For this review, take the finished solid that the model builds, in its own axes (mm). A direction names the side the tool comes from. Round coordinates to 2 decimals unless told otherwise and drop trailing zeros. Loops run counter-clockwise (first coordinate to the right, second up) from the corner with the lowest first, then second, coordinate; pieces in that order, holes last.
1) Take a section at D-D (y = 73.5). State the section outline as (x, z) points (3 decimals), then the cut area to 3 significant figures.
2) Take a section at A-A (y = 19). State the section outline as (x, z) points (3 decimals).
3) Take a section at B-B (x = -4). State the section outline as (y, z) points (3 decimals).
4) Mouldability with a two-part tool opening along Y and no side actions: class faces 4 (the flat face through (-31.75, -1, 283)), 5 (the flat face through (0.622, -246.174, -9.658)), 6 (the flat face through (1, 3, -9.525)), 7 (the flat face through (0.62, -240.94, -17.35)) as pulls with the +Y half, pulls with the -Y half, needs draft (parallel to the pull), parting line crosses it, or undercut.
5) Tool access review of faces 1 (the flat face through (0.622, 241.128, -17.574)), 2 (the flat face through (31.75, 1, 283)), 3 (the flat face through (0, 57.15, 275)): name each direction out of +Z, -Z, +X, -X, +Y, -Y from which nothing blocks a thin tool from reaching the whole face with its end or side.
6) Insertion check: pin 1 (10 mm diameter, centred on x = -3, z = 294, fed in from -Y); pin 2 (1.5 mm diameter, centred on y = 28, z = 144.5, fed in from -X); pin 3 (12 mm diameter, centred on x = -33, z = 262, fed in from +Y). Each pin has a flat end and moves straight along its axis. Give the tip position at first contact, or say it passes through.
7) Wall thickness on L1, parallel to Z at x = 18.5, y = -20 (3 decimals); L2, parallel to Z at x = -0.5, y = 86.5 (3 decimals); L3, parallel to X at y = 34, z = 45: over which ranges is each line inside the solid? List them lowest first.
8) Take a section at C-C (z = 388). State the section outline as (x, y) points.
```python
from build123d import *

# Parameters (mm, degrees)
F0_W      = 63.5
F0_H      = 114.3
F1_DEPTH  = 558.8
F2_SIZE   = 5.08
F4_DEPTH  = 25.4
F6_DEPTH  = 76.2
F8_DEPTH  = 12.7
F10_DEPTH = 12.7


with BuildPart() as f1:
    # F0 (on Top) → F1 (new body)
    with BuildSketch(Plane.XY):
        Rectangle(F0_W, F0_H)
    extrude(amount=F1_DEPTH)

    # F2
    f2_edges = [f1.edges().sort_by_distance(p)[0] for p in [
        (31.75, 57.15, 279.4),
        (-31.75, 57.15, 279.4),
        (-31.75, -57.15, 279.4),
        (31.75, -57.15, 279.4),
    ]]
    chamfer(f2_edges, length=F2_SIZE)

    # F3 (on face) → F4 (join)
    with BuildSketch(Plane(origin=(0, 0, 0), x_dir=(1, 0, 0), z_dir=(0, 0, -1))):
        Polygon((31.75, 52.07), (31.75, 254), (-31.75, 254), (-31.75, 52.07), (-26.67, 57.15), (26.67, 57.15), align=None)
        Polygon((31.75, -52.07), (31.75, 52.07), (26.67, 57.15), (-26.67, 57.15), (-31.75, 52.07), (-31.75, -52.07), (-26.67, -57.15), (26.67, -57.15), align=None)
        Polygon((31.75, -254), (31.75, -52.07), (26.67, -57.15), (-26.67, -57.15), (-31.75, -52.07), (-31.75, -254), align=None)
    extrude(amount=F4_DEPTH)

    # F5 (on face) → F6 (cut)
    with BuildSketch(Plane(origin=(-31.75, 0, 0), x_dir=(0, -1, 0), z_dir=(-1, 0, 0))):
        Polygon((238.125, 0), (254, -19.05), (254, 0), align=None)
        Polygon((-247.65, -25.4), (247.65, -25.4), (234.420833, -9.525), (-234.420833, -9.525), align=None)
        Polygon((-254, 0), (-254, -19.05), (-238.125, 0), align=None)
    extrude(amount=-F6_DEPTH, mode=Mode.SUBTRACT)

    # F7 (on face) → F8 (join)
    with BuildSketch(Plane.YZ.offset(31.75)):
        Polygon((238.125, 0), (52.07, 0), (-52.07, 0), (-238.125, 0), (-254, -19.05), (-254, -25.4), (-247.65, -25.4), (-234.420833, -9.525), (234.420833, -9.525), (247.65, -25.4), (254, -25.4), (254, -19.05), align=None)
    extrude(amount=F8_DEPTH)

    # F9 (on face) → F10 (join)
    with BuildSketch(Plane(origin=(-31.75, 0, 0), x_dir=(0, -1, 0), z_dir=(-1, 0, 0))):
        Polygon((238.125, 0), (52.07, 0), (-52.07, 0), (-238.125, 0), (-254, -19.05), (-254, -25.4), (-247.65, -25.4), (-234.420833, -9.525), (234.420833, -9.525), (247.65, -25.4), (254, -25.4), (254, -19.05), align=None)
    extrude(amount=F10_DEPTH)


solid = f1.part
```
Response:
1. outline: (-44.45, -9.525) - (44.45, -9.525) - (44.45, 0) - (-44.45, 0) - close
1. area: 847 mm2
2. outline: (-44.45, -9.525) - (44.45, -9.525) - (44.45, 0) - (31.75, 0) - (31.75, 558.8) - (-31.75, 558.8) - (-31.75, 0) - (-44.45, 0) - close
3. outline: (-254, -25.4) - (-247.65, -25.4) - (-234.421, -9.525) - (234.421, -9.525) - (247.65, -25.4) - (254, -25.4) - (254, -19.05) - (238.125, 0) - (57.15, 0) - (57.15, 558.8) - (-57.15, 558.8) - (-57.15, 0) - (-238.125, 0) - (-254, -19.05) - close
4. face 4: needs draft
4. face 5: pulls with the -Y half
4. face 6: undercut
4. face 7: undercut
5. face 1: -Z, +X, -X
5. face 2: +Z, +X, +Y, -Y
5. face 3: +Z, +X, -X, +Y
6. pin 1: stops at y = -57.15
6. pin 2: stops at x = -31.75
6. pin 3: stops at y = 56.82
7. L1: z = -9.525 to 558.8
7. L2: z = -9.525 to 0
7. L3: x = -31.75 to 31.75
8. outline: (-31.75, -52.07) - (-26.67, -57.15) - (26.67, -57.15) - (31.75, -52.07) - (31.75, 52.07) - (26.67, 57.15) - (-26.67, 57.15) - (-31.75, 52.07) - close
